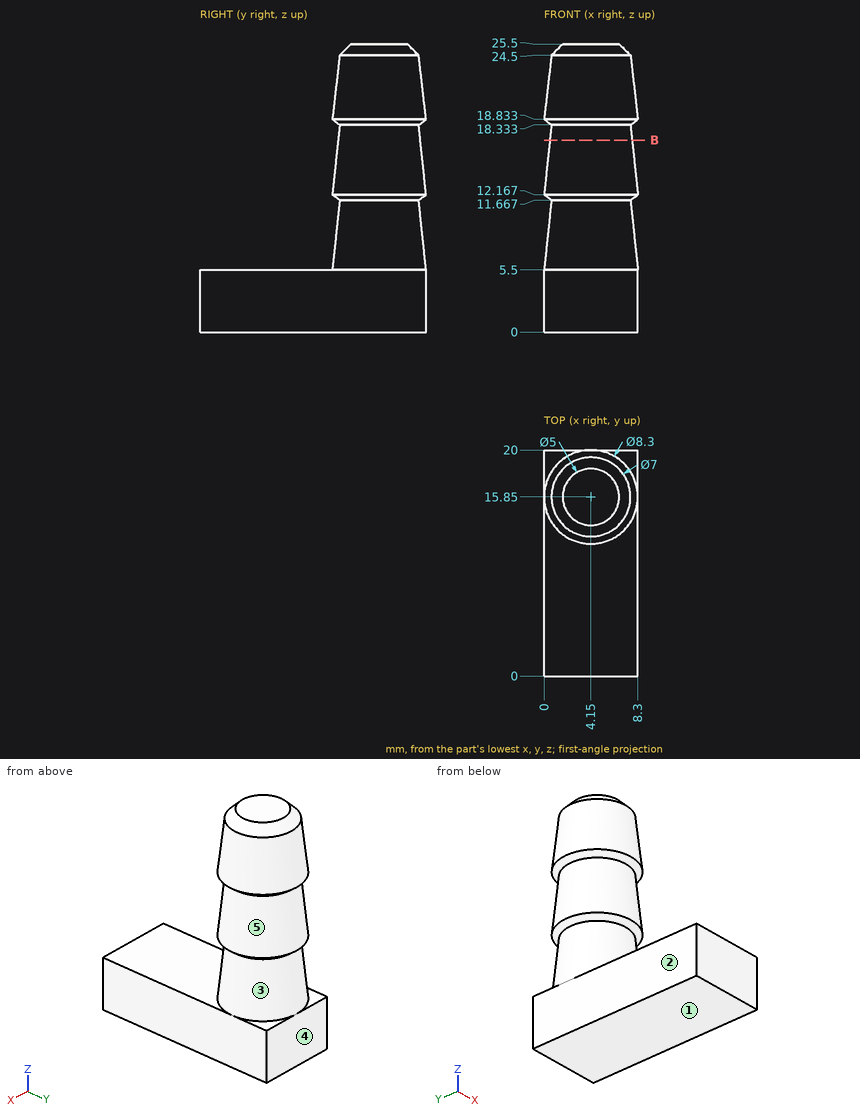
The drawing under review shows one solid part. Ordinate dimensions are in mm from its lowest x, y, z. A direction names the side the tool comes from. Round coordinates to 2 decimals unless told otherwise and drop trailing zeros. Loops run counter-clockwise (first coordinate to the right, second up) from the corner with the lowest first, then second, coordinate; pieces in that order, holes last.
Item 1: Take a section at B-B (z = 17). Write out the cut boundary in (x, y).
Determined:
outline: circle Ø7.28 at (4.15, 15.85)
Item 2: Mouldability with a two-part tool opening along Z and no side actions: class the marked faces 1, 2 and 3 as released by +Z, released by -Z, zero draft, split by the parting line, or undercut.
Determined:
face 1: released by -Z
face 2: zero draft
face 3: undercut
Item 3: Clearance check with flat-ended pins moving along their axes: pin 1 Ø1.2 at (x, y) = (7, 17.5) entering from +Z; pin 2 Ø2 at (x, y) = (7.5, 4.5) entering from +Z. State where each tip first meets the part, or that it passes through.
Determined:
pin 1: stops at z = 25.31
pin 2: stops at z = 5.5
Item 4: For the marked faces 4 and 5, list the 3-axis set-ups (+Z, -Z, +X, -X, +Y, -Y) from which the entire face can be reached by the end or side of a thin tool; tool diameter is ignored.
Determined:
face 4: +Z, -Z, +X, -X, +Y
face 5: none
Item 5: For line 1 (Z direction, x = 2.25, y = 2.5); line 2 (Y direction, x = 2, z = 15) (1 decimal); line 3 (Y direction, x = 0.75, z = 19) (1 decimal), list the stretches that pass through material, from the lowest coordinate up.
Determined:
line 1: z = 0 to 5.5
line 2: y = 12.7 to 19
line 3: y = 13.5 to 18.2
